For this review, take the finished solid that the model builds, in its own axes (mm). A direction names the side the tool comes from. Coordinates: 2 decimals unless noted, no trailing zeros. Order: outer loops, then holes, each group sorted by start corner. A loop starts at its lowest first (then second) coordinate and runs counter-clockwise, first axis right, second up. Notation, with made-up numbers: (60.5, 17) -> (68.5, 17) arc R25 ccw to (68.5, 56) -> close; hole circle Ø4 at (37.25, 49). An arc over 180 degrees is marked (long way). Return JSON: item names as keys, results as strings. Group by question number.
Item 1: Take a section at B-B (z = 1074). Write out the cut boundary in (x, y) (3 decimals).
Item 2: Insertion check: pin 1 (1.6 mm diameter, centred on x = 7.5, y = 1.5, fed in from +Z); pin 2 (4 mm diameter, centred on x = 9.5, z = 1163.5, fed in from +Y) (3 decimals); pin 3 (5.5 mm diameter, centred on y = 12.7, z = 1184.98, fed in from +X) (3 decimals). Each pin has a flat end and moves straight along its axis. Give the tip position at first contact, or say it passes through.
Item 3: For line 1 along Z through (x, y) = (1, 12.7); line 2 along X through (y, z) = (1.15, 1099.2) (3 decimals); line 3 along Z through (x, y) = (9.5, 1), list the stretches that pass through material, from the lowest coordinate up.
Item 4: Take a section at C-C (x = 7.25). Write out the cut boundary in (y, z) (3 decimals).
Item 5: Draft analysis for pull direction Y (two halves, no side actions). For faces 1 (the cylindrical face through (12.178, 1.61, 1181.897)), 2 (the cylindrical face through (1.61, 12.342, 1051.815)), 3 (the cylindrical face through (1.61, 10.46, 1170.836)), 4 (the flat face through (2, 25.4, 1121)), state which applies: +Y half, -Y half, draft (parallel to the pull), parting line (faces both ways), or undercut.
Item 6: Take a section at D-D (y = 18.5). Write out the cut boundary in (x, z) (3 decimals).
Item 7: Machinability: for faces 5 (the flat face through (2, 3.175, 1208)), 6 (the flat face through (2, 3.175, 1030)), 7 (the flat face through (0, 13, 1121)), which of the approach directions +Z, -Z, +X, -X, +Y, -Y give a long, thin tool a straight path to every point of the face, cutting with its end or side? Answer none if there is none.
Item 8: Take a section at A-A (z = 1129.2). Write out the cut boundary in (x, y) (3 decimals).
```python
from build123d import *

# Parameters (mm, degrees)
BOSS_EXTRUDE1_DEPTH = 1219.2
FILLET1_R           = 0.4064
SKETCH4_W           = 2238.4
SKETCH4_H           = 103.278519729
CUT_EXTRUDE1_DEPTH  = 60
SKETCH5_W           = 25.4
SKETCH5_H           = 22.23
CUT_EXTRUDE2_DEPTH  = 3.175
SKETCH6_W           = 25.4
SKETCH6_H           = 22.23
CUT_EXTRUDE3_DEPTH  = 3.175
SKETCH7_W           = 1.26890891
SKETCH7_H           = 1.024965533
CUT_EXTRUDE4_DEPTH  = 220
SKETCH9_R           = 1.65
CUT_EXTRUDE5_DEPTH  = 20
SKETCH10_R          = 1.65
CUT_EXTRUDE6_DEPTH  = 20
SKETCH11_R          = 1.65
CUT_EXTRUDE7_DEPTH  = 70
SKETCH12_R          = 1.65
CUT_EXTRUDE8_DEPTH  = 70


with BuildPart() as part:
    # Sketch3 → Boss-Extrude1 (new, symmetric)
    with BuildSketch(Plane.XY):
        Polygon((3.175, 25.4), (0, 25.4), (0, 0), (25.4, 0), (25.4, 3.175), (3.175, 3.175), align=None)
    extrude(amount=BOSS_EXTRUDE1_DEPTH, both=True)

    # Fillet1
    fillet1_edges = [part.edges().sort_by_distance(p)[0] for p in [
        (3.175, 3.175, 0),
    ]]
    fillet(fillet1_edges, radius=FILLET1_R)

    # Sketch4 → Cut-Extrude1 (cut)
    with BuildSketch(Plane.ZY):
        with Locations((-100, -26.239259864)):
            Rectangle(SKETCH4_W, SKETCH4_H)
    extrude(amount=-CUT_EXTRUDE1_DEPTH, mode=Mode.SUBTRACT)

    # Sketch5 → Cut-Extrude2 (cut)
    with BuildSketch(Plane.XZ):
        with Locations((12.7, 1030.315)):
            Rectangle(SKETCH5_W, SKETCH5_H)
    extrude(amount=-CUT_EXTRUDE2_DEPTH, mode=Mode.SUBTRACT)

    # Sketch6 → Cut-Extrude3 (cut)
    with BuildSketch(Plane.XZ):
        with Locations((12.7, 1208.085)):
            Rectangle(SKETCH6_W, SKETCH6_H)
    extrude(amount=-CUT_EXTRUDE3_DEPTH, mode=Mode.SUBTRACT)

    # Sketch7 → Cut-Extrude4 (cut)
    with BuildSketch(Plane(origin=(0, 0, 1019.2), x_dir=(-1, 0, 0), z_dir=(0, 0, -1))):
        with Locations((-3.809454455, 3.687482767)):
            Rectangle(SKETCH7_W, SKETCH7_H)
    extrude(amount=-CUT_EXTRUDE4_DEPTH, mode=Mode.SUBTRACT)

    # Sketch9 → Cut-Extrude5 (cut)
    with BuildSketch(Plane(origin=(3.175, 0, 0), x_dir=(0, 0, -1), z_dir=(1, 0, 0))):
        with Locations(Location((-1169.2, 10.675, 0), (0, 0, 90))):
            Circle(SKETCH9_R)
        with Locations(Location((-1149.2, 10.675, 0), (0, 0, 90))):
            Circle(SKETCH9_R)
        with Locations(Location((-1129.2, 10.675, 0), (0, 0, 90))):
            Circle(SKETCH9_R)
        with Locations(Location((-1109.2, 10.675, 0), (0, 0, 90))):
            Circle(SKETCH9_R)
        with Locations(Location((-1089.2, 10.675, 0), (0, 0, 90))):
            Circle(SKETCH9_R)
        with Locations(Location((-1069.2, 10.675, 0), (0, 0, 90))):
            Circle(SKETCH9_R)
    extrude(amount=-CUT_EXTRUDE5_DEPTH, mode=Mode.SUBTRACT)

    # Sketch10 → Cut-Extrude6 (cut)
    with BuildSketch(Plane(origin=(0, 3.175, 0), x_dir=(1, 0, 0), z_dir=(0, 1, 0))):
        with Locations(Location((10.675, -1079.2, 0), (0, 0, 180))):
            Circle(SKETCH10_R)
        with Locations(Location((10.675, -1099.2, 0), (0, 0, 180))):
            Circle(SKETCH10_R)
        with Locations(Location((10.675, -1119.2, 0), (0, 0, 180))):
            Circle(SKETCH10_R)
        with Locations(Location((10.675, -1139.2, 0), (0, 0, 180))):
            Circle(SKETCH10_R)
        with Locations(Location((10.675, -1159.2, 0), (0, 0, 180))):
            Circle(SKETCH10_R)
    extrude(amount=-CUT_EXTRUDE6_DEPTH, mode=Mode.SUBTRACT)

    # Sketch11 → Cut-Extrude7 (cut)
    with BuildSketch(Plane(origin=(3.175, 0, 0), x_dir=(0, 0, -1), z_dir=(1, 0, 0))):
        with Locations(Location((-1053.425704333, 12.7, 0), (0, 0, 90))):
            Circle(SKETCH11_R)
        with Locations(Location((-1184.979295667, 12.7, 0), (0, 0, 90))):
            Circle(SKETCH11_R)
    extrude(amount=-CUT_EXTRUDE7_DEPTH, mode=Mode.SUBTRACT)

    # Sketch12 → Cut-Extrude8 (cut)
    with BuildSketch(Plane(origin=(0, 3.175, 0), x_dir=(1, 0, 0), z_dir=(0, 1, 0))):
        with Locations(Location((11.9634, -1180.260622857, 0), (0, 0, 180))):
            Circle(SKETCH12_R)
        with Locations(Location((11.9634, -1060.48, 0), (0, 0, 180))):
            Circle(SKETCH12_R)
    extrude(amount=-CUT_EXTRUDE8_DEPTH, mode=Mode.SUBTRACT)


solid = part.part
```
Findings below:
{
 "1": {"outline": "(0, 0) -> (25.4, 0) -> (25.4, 3.175) -> (3.175, 3.175) -> (3.175, 25.4) -> (0, 25.4) -> close"},
 "2": {"pin 1": "stops at z = 1196.97", "pin 2": "stops at y = 3.175", "pin 3": "stops at x = 3.175"},
 "3": {"line 1": "z = 1019.2 to 1051.78, 1055.08 to 1183.33, 1186.63 to 1219.2", "line 2": "x = 0 to 9.025, 12.325 to 25.4", "line 3": "z = 1041.43 to 1078.04, 1080.36 to 1098.04, 1100.36 to 1118.04, 1120.36 to 1138.04, 1140.36 to 1158.04, 1160.36 to 1196.97"},
 "4": {"outline": "(0, 1041.43) -> (3.175, 1041.43) -> (3.175, 1196.97) -> (0, 1196.97) -> close"},
 "5": {"face 1": "draft", "face 2": "undercut", "face 3": "undercut", "face 4": "+Y half"},
 "6": {"outline": "(0, 1019.2) -> (3.175, 1019.2) -> (3.175, 1219.2) -> (0, 1219.2) -> close"},
 "7": {"face 5": "+Z, +X, -X, -Y", "face 6": "-Z, +X, -X, -Y", "face 7": "+Z, -Z, -X, +Y, -Y"},
 "8": {"outline": "(0, 0) -> (25.4, 0) -> (25.4, 3.175) -> (3.175, 3.175) -> (3.175, 9.025) -> (0, 9.025) -> close; (0, 12.325) -> (3.175, 12.325) -> (3.175, 25.4) -> (0, 25.4) -> close"}
}
